Design review of the part built by this model. Coordinates are the model's own, in mm. Face numbers are marked on the shaded views. Coordinates: 2 decimals unless noted, no trailing zeros. Loops run counter-clockwise (first coordinate to the right, second up) from the corner with the lowest first, then second, coordinate; pieces in that order, holes last.
Q1. Add section D-D on x = 58. Give the boundary of the cut face in (y, z), and give its area (3 significant figures).
Q2. Draft analysis for pull direction Y (two halves, no side actions). For the marked faces 1, 2 and 3, state which applies: released by +Y, released by -Y, zero draft, split by the parting line, or undercut.
Q3. For P1, Ø21, axis at y = 137.5, z = -8.5, coming from the -X side; P2, Ø25, axis at x = 99, y = -34.5, coming from the -Z side; P3, Ø10, axis at x = -13, z = -46, coming from the -Y side, all flat-tipped, find the tip position at first contact; note any pin that passes through.
Q4. Add section C-C on x = -13.5. Give the boundary of the cut face in (y, z), and give its area (3 significant figures).
Q5. Wall thickness on probe 1 along Z at (x, y) = (-9.5, 93); probe 2 along Y at (x, z) = (-34.5, -104.5); probe 3 along Z at (x, y) = (52, 74): over which ranges is each line inside the solid? List them lowest first.
Q6. Add section A-A on z = 90. Give the boundary of the cut face in (x, y).
Q7. Add section B-B on y = 92.5. Give the boundary of the cut face in (x, z), and give its area (3 significant figures).
```python
from build123d import *

# Parameters (mm, degrees)
F0_W      = 140
F0_H      = 150
F1_DEPTH  = 20
F2_DEPTH  = 25
F4_DEPTH  = 19
F5_W      = 20
F5_H      = 10.7958046891
F6_DEPTH  = 146
F7_W      = 32.1311553568
F7_H      = 22.5257221609
F8_DEPTH  = 125
F9_W      = 20
F9_H      = 8.2833381355
F10_DEPTH = 228


with BuildPart() as f1:
    # F0 (on Top) → F1 (new body)
    with BuildSketch(Plane.XY):
        with Locations((43.1068145484, 28.9318494499)):
            Rectangle(F0_W, F0_H)
    extrude(amount=F1_DEPTH)

    # F2 (add): a face of the model
    f2_faces = [f1.faces().sort_by_distance(p)[0] for p in [
        (43.1068145484, 103.9318494499, 10),
    ]]
    extrude(f2_faces, amount=F2_DEPTH)

    # F3 (on face) → F4 (join)
    with BuildSketch(Plane(origin=(0, 128.9318494499, 0), x_dir=(-1, 0, 0), z_dir=(0, 1, 0))):
        Polygon((6.8931854516, 101.1020294233), (26.8931854516, 101.1020294233), (26.8931854516, 142.6936388016), (-113.1068145484, 142.6936388016), (-113.1068145484, -122.8044226003), (43.6474412288, -122.8044226003), (43.6474412288, -102.8044226003), (-93.1068145484, -102.8044226003), (-93.1068145484, 122.6936388016), (6.8931854516, 122.6936388016), align=None)
    extrude(amount=F4_DEPTH)

    # F5 (on face) → F6 (join)
    with BuildSketch(Plane.XZ.offset(-128.9318494499)):
        with Locations((-16.8931854516, 106.4999317679)):
            Rectangle(F5_W, F5_H)
    extrude(amount=F6_DEPTH)

    # F7 (on face) → F8 (join)
    with BuildSketch(Plane(origin=(0, 0, 0), x_dir=(1, 0, 0), z_dir=(0, 0, -1))):
        with Locations((97.04123687, 34.8052894697)):
            Rectangle(F7_W, F7_H)
    extrude(amount=F8_DEPTH)

    # F9 (on face) → F10 (join)
    with BuildSketch(Plane(origin=(0, 0, 101.1020294233), x_dir=(1, 0, 0), z_dir=(0, 0, -1))):
        with Locations((-16.8931854516, 12.9264814824)):
            Rectangle(F9_W, F9_H)
    extrude(amount=F10_DEPTH)


solid = f1.part
```
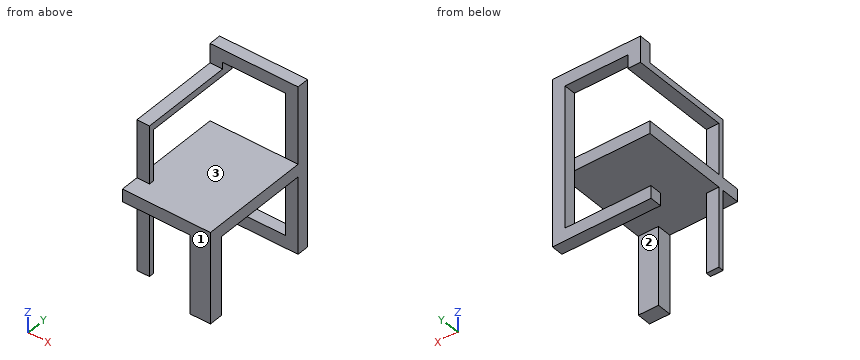
Entries:
1. outline: (-46.07, 0) - (128.93, 0) - (128.93, 20) - (-46.07, 20) - close; (128.93, -122.8) - (147.93, -122.8) - (147.93, -102.8) - (128.93, -102.8) - close; (128.93, 122.69) - (147.93, 122.69) - (147.93, 142.69) - (128.93, 142.69) - close
1. area: 4,260 mm2
2. face 1: released by -Y
2. face 2: undercut
2. face 3: zero draft
3. P1: stops at x = 93.11
3. P2: stops at z = -125
3. P3: stops at y = -17.07
4. outline: (-46.07, 0) - (-17.07, 0) - (-17.07, -126.9) - (-8.78, -126.9) - (-8.78, 0) - (128.93, 0) - (128.93, 20) - (-8.78, 20) - (-8.78, 101.1) - (147.93, 101.1) - (147.93, 142.69) - (128.93, 142.69) - (128.93, 111.9) - (-17.07, 111.9) - (-17.07, 20) - (-46.07, 20) - close; (128.93, -122.8) - (147.93, -122.8) - (147.93, -102.8) - (128.93, -102.8) - close
4. area: 7,970 mm2
5. probe 1: z = 0 to 20, 101.1 to 111.9
5. probe 2: y = 128.93 to 147.93
5. probe 3: z = 0 to 20
6. outline: (-26.89, -17.07) - (-6.89, -17.07) - (-6.89, -8.78) - (-26.89, -8.78) - close; (93.11, 128.93) - (113.11, 128.93) - (113.11, 147.93) - (93.11, 147.93) - close
7. outline: (-26.89, 0) - (113.11, 0) - (113.11, 20) - (-26.89, 20) - close; (-26.89, 101.1) - (-6.89, 101.1) - (-6.89, 111.9) - (-26.89, 111.9) - close
7. area: 3,020 mm2
